The model under review builds one solid part; all positions refer to its coordinate system, in mm. A direction names the side the tool comes from. Round coordinates to 2 decimals unless told otherwise and drop trailing zeros. Write each loop counter-clockwise with the first axis right and the second up, starting at its lowest first coordinate (ties: lowest second). Pieces come first, ordered by that corner, then holes. Notation, with made-up numbers: (-24.5, 61) -> (0.5, 61) arc R25 ccw to (0.5, 92) -> close; hole circle Ø4 at (86, 22). An arc over 180 degrees is marked (long way). Return JSON: item names as keys, results as strings. Group by question number.
1. Tool access review of faces 4 (the flat face through (-165, 5, -215)), 5 (the flat face through (-165, -5, 215)), 6 (the flat face through (-165, -15, -3)), 7 (the flat face through (-165, -10, -200)), 8 (the flat face through (-165, 5, 215)): name each direction out of +Z, -Z, +X, -X, +Y, -Y from which nothing blocks a thin tool from reaching the whole face with its end or side.
2. Mouldability with a two-part tool opening along Z and no side actions: class faces 1 (the flat face through (-165, 10, -200)), 2 (the flat face through (-165, 15, -3)), 3 (the flat face through (-165, -10, 200)) as pulls with the +Z half, pulls with the -Z half, needs draft (parallel to the pull), parting line crosses it, or undercut.
3. Clearance check with flat-ended pins moving along their axes: P1, Ø8, axis at x = -162.5, y = 9.5, coming from the -Z side; P2, Ø15, axis at x = -159, z = 216, coming from the +Y side; P3, Ø9, axis at x = -171.5, z = 214, coming from the -Y side. State where each tip first meets the part, or that it passes through.
4. Take a section at B-B, the plane y = -9. Write out the cut boundary in (x, z).
5. Take a section at A-A, the plane x = -156. Write out the cut boundary in (y, z).
6. For line 1 along Z through (x, y) = (-159, 9.75), list the stretches that pass through material, from the lowest coordinate up. Write a range as from..to.
from build123d import *

# Parameters (mm, degrees)
CROQUIS1_W              = 29.994038168
CROQUIS1_H              = 460
SALIENTE_EXTRUIR1_DEPTH = 5
CROQUIS2_W              = 29.994038168
CROQUIS2_H              = 400
SALIENTE_EXTRUIR2_DEPTH = 15


with BuildPart() as part:
    # Croquis1 → Saliente-Extruir1 (new, symmetric)
    with BuildSketch(Plane(origin=(0, 0, 0), x_dir=(1, 0, 0), z_dir=(0, 1, 0))):
        with Locations((-165, 0)):
            Rectangle(CROQUIS1_W, CROQUIS1_H)
    extrude(amount=SALIENTE_EXTRUIR1_DEPTH, both=True)

    # Croquis2 → Saliente-Extruir2 (add, symmetric)
    with BuildSketch(Plane(origin=(0, 0, 0), x_dir=(1, 0, 0), z_dir=(0, 1, 0))):
        with Locations((-165, 0)):
            Rectangle(CROQUIS2_W, CROQUIS2_H)
    extrude(amount=SALIENTE_EXTRUIR2_DEPTH, both=True)


solid = part.part
Output:
{
 "1": {"face 4": "-Z, +X, -X, +Y", "face 5": "+Z, +X, -X, -Y", "face 6": "+Z, -Z, +X, -X, -Y", "face 7": "-Z, +X, -X, -Y", "face 8": "+Z, +X, -X, +Y"},
 "2": {"face 1": "pulls with the -Z half", "face 2": "needs draft", "face 3": "pulls with the +Z half"},
 "3": {"P1": "stops at z = -200", "P2": "stops at y = 5", "P3": "stops at y = -5"},
 "4": {"outline": "(-180, -200) -> (-150, -200) -> (-150, 200) -> (-180, 200) -> close"},
 "5": {"outline": "(-15, -200) -> (-5, -200) -> (-5, -230) -> (5, -230) -> (5, -200) -> (15, -200) -> (15, 200) -> (5, 200) -> (5, 230) -> (-5, 230) -> (-5, 200) -> (-15, 200) -> close"},
 "6": {"line 1": "z = -200..200"}
}
